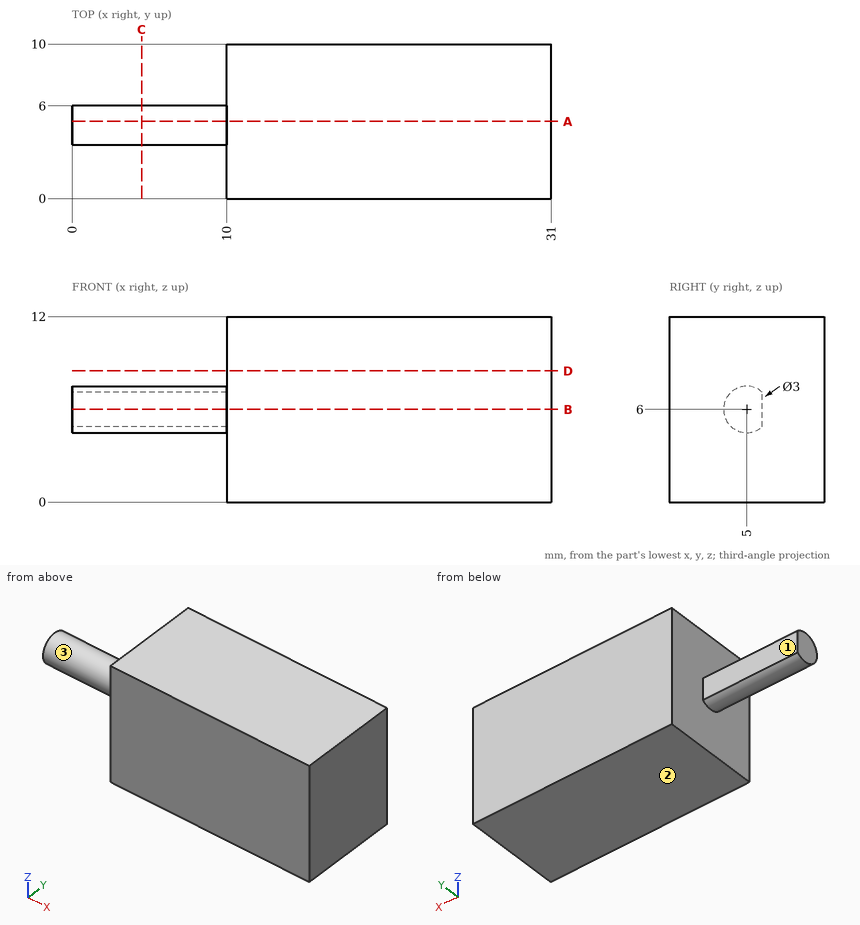
Verification items for this drawing (mm, ordinates from the low corner). A direction names the side the tool comes from. Give positions to 0.01 mm unless a question says otherwise; leave off trailing zeros. Order: outer loops, then holes, each group sorted by start corner. A loop starts at its lowest first (then second) coordinate and runs counter-clockwise, first axis right, second up. Notation, with made-up numbers: M 15,45 L 64,45 A8 ccw 64,52 Z; hole C 76,48.25 d1. An arc over 180 degrees is marked long. Use a Markdown table: item, result.
Item 1: Section check D-D (z = 8.5). Record the cut outline in (x, y).
Answers follow:
| item | result |
|---|---|
| outline | M 10,0 L 31,0 L 31,10 L 10,10 Z |
Item 2: Section check A-A (y = 5). Record the cut outline in (x, z).
Answers follow:
| item | result |
|---|---|
| outline | M 0,4.5 L 10,4.5 L 10,0 L 31,0 L 31,12 L 10,12 L 10,7.5 L 0,7.5 Z |
Item 3: Section check C-C (x = 4.5). Record the cut outline in (y, z), and give its area (3 significant figures).
Answers follow:
| item | result |
|---|---|
| outline | M 6,4.88 L 6,7.12 A1.5 ccw long Z |
| area | 6.29 mm2 |
Item 4: Material ranges on line 1 along X through (y, z) = (5.25, 3); line 2 along Y through (x, z) = (3.5, 5); line 3 along Y through (x, z) = (5, 6.75), recorded low to high.
Answers follow:
| item | result |
|---|---|
| line 1 | x = 10 to 31 |
| line 2 | y = 3.88 to 6 |
| line 3 | y = 3.7 to 6 |
Item 5: Depth check by flat-ended pin: P1, Ø5, axis at x = 6, y = 1.5, coming from the +Z side; P2, Ø5, axis at y = 7, z = 2, coming from the -X side; P3, Ø1.8, axis at x = 6.5, z = 5.5, coming from the +Y side. Enter the tip coordinate at first touch or a pass-through.
Answers follow:
| item | result |
|---|---|
| P1 | stops at z = 7.12 |
| P2 | stops at x = 10 |
| P3 | stops at y = 6 |
Item 6: Tool access check on the marked faces 1, 2 and 3. Record the directions out of +Z, -Z, +X, -X, +Y, -Y that give a thin tool (end or side, any length) a straight path to the whole face; none if there is none.
Answers follow:
| item | result |
|---|---|
| face 1 | +Z, -Z, -X, +Y |
| face 2 | -Z, +X, -X, +Y, -Y |
| face 3 | -X |
Item 7: Section check B-B (z = 6). Record the cut outline in (x, y).
Answers follow:
| item | result |
|---|---|
| outline | M 0,3.5 L 10,3.5 L 10,0 L 31,0 L 31,10 L 10,10 L 10,6 L 0,6 Z |
